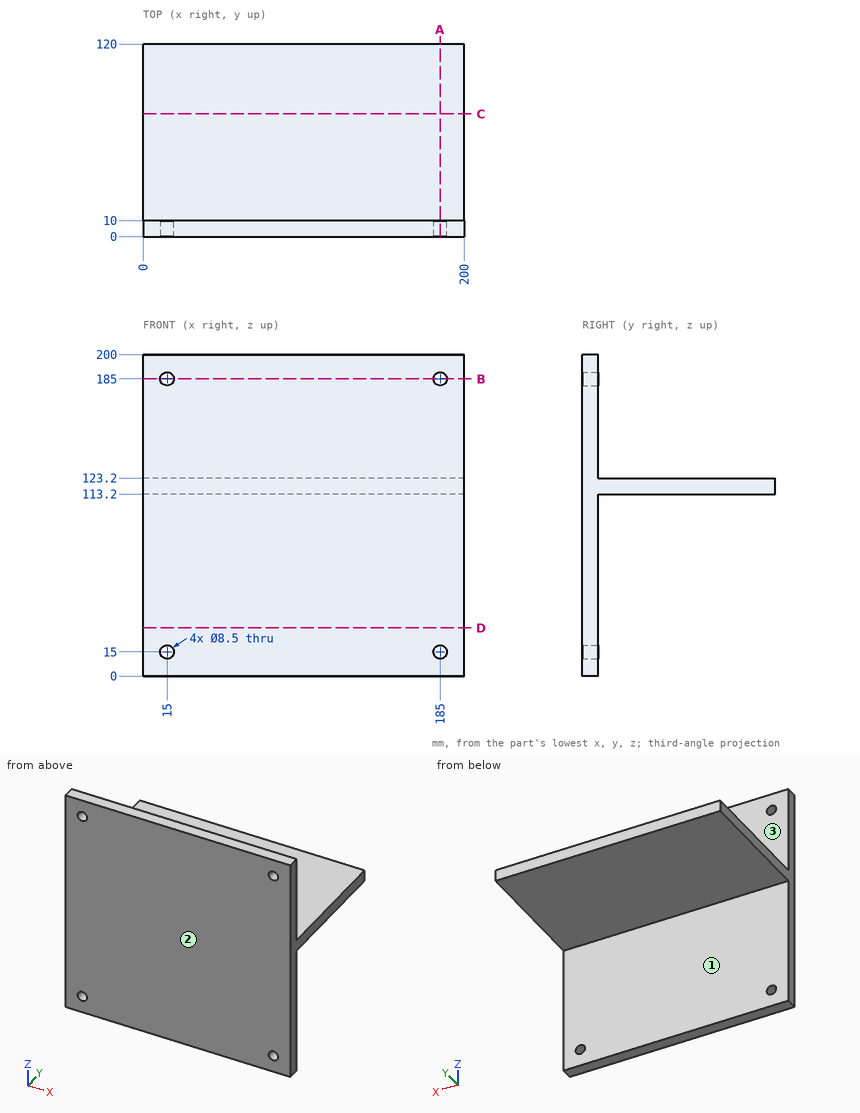
Job drawing, mm, ordinate dimensions from the low corner. One solid piece. A direction names the side the tool comes from. Coordinates: 2 decimals unless noted, no trailing zeros. Order: outer loops, then holes, each group sorted by start corner. A loop starts at its lowest first (then second) coordinate and runs counter-clockwise, first axis right, second up. Notation, with made-up numbers: (20, 67) -> (63, 67) arc R23 ccw to (63, 94) -> close; hole circle Ø3 at (28.5, -28). An arc over 180 degrees is marked (long way). Answer in a Markdown table with one row per item. Add a question column.
Q1. Band-saw the part on A-A, the plane x = 185. List the corners of the cut face in (y, z), then the cut area to 3 significant figures.
Q2. Band-saw the part on C-C, the plane y = 76.5. List the corners of the cut face in (x, z), then the cut area to 3 significant figures.
Q3. Wall check: line 1 along Z through (x, y) = (15, 6); line 2 along Z through (x, y) = (187, 7.5). Give the ranges that are in metal, low to high. Write a range as [from, to].
Q4. Band-saw the part on D-D, the plane z = 30. List the corners of the cut face in (x, y), then the cut area to 3 significant figures.
Q5. Drop flat-ended pins along their axis: pin 1 (23 mm diameter, centred on x = 51, z = 180, fed in from +Y); pin 2 (1.5 mm diameter, centred on x = 99, y = 26, fed in from -Z); pin 3 (10 mm diameter, centred on x = 101, y = 88, fed in from +Z). Give the stop position or say it passes through.
Q6. Which spindle directions (+Z, -Z, +X, -X, +Y, -Y) get a long thin tool onto all of the face, cutting with end or side? Do the marked faces 1, 2 and 3. Say none if no direction does.
Q7. Band-saw the part on B-B, the plane z = 185. List the corners of the cut face in (x, y), then the cut area to 3 significant figures.
Answers follow:
| question | item | result |
|---|---|---|
| 1 | outline | (0, 0) -> (10, 0) -> (10, 10.75) -> (0, 10.75) -> close; (0, 19.25) -> (10, 19.25) -> (10, 113.2) -> (120, 113.2) -> (120, 123.2) -> (10, 123.2) -> (10, 180.75) -> (0, 180.75) -> close; (0, 189.25) -> (10, 189.25) -> (10, 200) -> (0, 200) -> close |
| 1 | area | 2,930 mm^2 |
| 2 | outline | (0, 113.2) -> (200, 113.2) -> (200, 123.2) -> (0, 123.2) -> close |
| 2 | area | 2,000 mm^2 |
| 3 | line 1 | [0, 10.75], [19.25, 180.75], [189.25, 200] |
| 3 | line 2 | [0, 11.25], [18.75, 181.25], [188.75, 200] |
| 4 | outline | (0, 0) -> (200, 0) -> (200, 10) -> (0, 10) -> close |
| 4 | area | 2,000 mm^2 |
| 5 | pin 1 | y = 10 |
| 5 | pin 2 | z = 113.2 |
| 5 | pin 3 | z = 123.2 |
| 6 | face 1 | -Z, +X, -X, +Y |
| 6 | face 2 | +Z, -Z, +X, -X, -Y |
| 6 | face 3 | +Z, +X, -X, +Y |
| 7 | outline | (0, 0) -> (10.75, 0) -> (10.75, 10) -> (0, 10) -> close; (19.25, 0) -> (180.75, 0) -> (180.75, 10) -> (19.25, 10) -> close; (189.25, 0) -> (200, 0) -> (200, 10) -> (189.25, 10) -> close |
| 7 | area | 1,830 mm^2 |
